from build123d import *

# Parameters (mm, degrees)
F1_DEPTH = 2
F0_W     = 28.0000002682
F0_H     = 45
F0_H_2   = 2
F0_W_2   = 23
F0_W_3   = 4.9999997318
F0_W_4   = 5
F2_DEPTH = 2
F3_DEPTH = 12


with BuildPart() as f1:
    # F0 (on Top) → F1 (new body)
    with BuildSketch(Plane.XY):
        Polygon((-18, 22.5), (-43, 22.5), (-43, -17.5), (-43, -22.5), (-18, -22.5), align=None)
        Polygon((-18, -24.5), (-18, -22.5), (-43, -22.5), (-45, -22.5), (-45, -24.5), align=None)
        Polygon((-43, -17.5), (-43, 22.5), (-18, 22.5), (-18, 24.5), (-45, 24.5), (-45, -17.5), align=None)
    extrude(amount=-F1_DEPTH)



with BuildPart() as f1b:
    # F0 (on Top) → F1, piece 2 (new body)
    with BuildSketch(Plane.XY):
        with Locations((0.9999998659, 0)):
            Rectangle(F0_W, F0_H)
        with Locations((0.9999998659, -23.5)):
            Rectangle(F0_W, F0_H_2)
        with Locations((0.9999998659, 23.5)):
            Rectangle(F0_W, F0_H_2)
    extrude(amount=-F1_DEPTH)


with BuildPart() as f1c:
    # F0 (on Top) → F1, piece 3 (new body)
    with BuildSketch(Plane.XY):
        with Locations((31.5, 0)):
            Rectangle(F0_W_2, F0_H)
        Polygon((20, 24.5), (20, 22.5), (43, 22.5), (43, -22.5), (20, -22.5), (20, -24.5), (45, -24.5), (45, 24.5), align=None)
    extrude(amount=-F1_DEPTH)


with BuildPart() as f1_1:
    add(f1.part)

    add(f1b.part)  # F2 merges F1b

    add(f1c.part)  # F2 merges F1c
    # F0 (on Top) → F2 (join)
    with BuildSketch(Plane.XY):
        with Locations((31.5, 0)):
            Rectangle(F0_W_2, F0_H)
        with Locations((0.9999998659, 0)):
            Rectangle(F0_W, F0_H)
        Polygon((-18, 22.5), (-43, 22.5), (-43, -17.5), (-43, -22.5), (-18, -22.5), align=None)
        with Locations((-15.5000001341, 0)):
            Rectangle(F0_W_3, F0_H)
        with Locations((17.5, 0)):
            Rectangle(F0_W_4, F0_H)
    extrude(amount=F2_DEPTH)

    # F0 (on Top) → F3 (join)
    with BuildSketch(Plane.XY):
        Polygon((-43, -17.5), (-43, 22.5), (-18, 22.5), (-18, 24.5), (-45, 24.5), (-45, -17.5), align=None)
        Polygon((-18, -24.5), (-18, -22.5), (-43, -22.5), (-45, -22.5), (-45, -24.5), align=None)
        with Locations((0.9999998659, -23.5)):
            Rectangle(F0_W, F0_H_2)
        with Locations((0.9999998659, 23.5)):
            Rectangle(F0_W, F0_H_2)
        Polygon((20, 24.5), (20, 22.5), (43, 22.5), (43, -22.5), (20, -22.5), (20, -24.5), (45, -24.5), (45, 24.5), align=None)
    extrude(amount=F3_DEPTH)


solid = f1_1.part
Verification items for the finished model (mm, model axes). A direction names the side the tool comes from. Coordinates: 2 decimals unless noted, no trailing zeros. Loops run counter-clockwise (first coordinate to the right, second up) from the corner with the lowest first, then second, coordinate; pieces in that order, holes last. Notation, with made-up numbers: (-24.5, -33.5) -> (22.5, -33.5) arc R21 cw to (22.5, 1.5) -> close; hole circle Ø4 at (-31, 69.5). An arc over 180 degrees is marked (long way). Answer as CSV lines item,"result".
1) Cross-section at C-C, the plane x = -23.5. Record the cut outline in (y, z).
Found:
outline,"(-24.5, -2) -> (24.5, -2) -> (24.5, 12) -> (22.5, 12) -> (22.5, 2) -> (-22.5, 2) -> (-22.5, 12) -> (-24.5, 12) -> close"
2) Thickness scan on L1, parallel to Y at x = -28.5, z = 4.5; L2, parallel to X at y = 17, z = 4.25; L3, parallel to Z at x = -3, y = -8. Record the ranges inside material, lowest first. Write a range as from..to.
Found:
L1,"y = -24.5..-22.5, 22.5..24.5"
L2,"x = -45..-43, 43..45"
L3,"z = -2..2"
3) Cross-section at D-D, the plane y = 11. Record the cut outline in (x, z).
Found:
outline,"(-45, -2) -> (-18, -2) -> (-18, 0) -> (-13, 0) -> (-13, -2) -> (15, -2) -> (15, 0) -> (20, 0) -> (20, -2) -> (45, -2) -> (45, 12) -> (43, 12) -> (43, 2) -> (-43, 2) -> (-43, 12) -> (-45, 12) -> close"
4) Cross-section at A-A, the plane z = 9.25. Record the cut outline in (x, y).
Found:
outline,"(-45, -24.5) -> (-18, -24.5) -> (-18, -22.5) -> (-45, -22.5) -> close; (-45, -17.5) -> (-43, -17.5) -> (-43, 22.5) -> (-18, 22.5) -> (-18, 24.5) -> (-45, 24.5) -> close; (-13, -24.5) -> (15, -24.5) -> (15, -22.5) -> (-13, -22.5) -> close; (-13, 22.5) -> (15, 22.5) -> (15, 24.5) -> (-13, 24.5) -> close; (20, -24.5) -> (45, -24.5) -> (45, 24.5) -> (20, 24.5) -> (20, 22.5) -> (43, 22.5) -> (43, -22.5) -> (20, -22.5) -> close"
5) Release check for a two-part mould opening along X. For faces 1 (the flat face through (-1, 0, 2)), 2 (the flat face through (-32, -23, 12)), 3 (the flat face through (-45, 4, 5)) record: +X half, -X half, draft (parallel to the pull), parting line (faces both ways), or undercut.
Found:
face 1,"undercut"
face 2,"draft"
face 3,"-X half"
6) Depth check by flat-ended pin: pin 1 (1 mm diameter, centred on x = -15.5, z = 0.5, fed in from -Y); pin 2 (3 mm diameter, centred on x = 34, y = -14, fed in from +Z); pin 3 (1.5 mm diameter, centred on x = 18, y = 4, fed in from -Z). Enter the tip coordinate at first touch or a pass-through.
Found:
pin 1,"stops at y = -22.5"
pin 2,"stops at z = 2"
pin 3,"stops at z = 0"
7) Cross-section at B-B, the plane y = -19. Record the cut outline in (x, z).
Found:
outline,"(-43, -2) -> (-18, -2) -> (-18, 0) -> (-13, 0) -> (-13, -2) -> (15, -2) -> (15, 0) -> (20, 0) -> (20, -2) -> (45, -2) -> (45, 12) -> (43, 12) -> (43, 2) -> (-43, 2) -> close"
8) Tool access check on faces 4 (the flat face through (-16, -22.5, 1)), 5 (the flat face through (-31, -22.5, 6)), 6 (the flat face through (-31, 22.5, 7)). Record the directions out of +Z, -Z, +X, -X, +Y, -Y that give a thin tool (end or side, any length) a straight path to the whole face; none if there is none.
Found:
face 4,"+Z, -Z, -Y"
face 5,"+Z, -X"
face 6,"+Z"
